Verification items for the finished model (mm, model axes). A direction names the side the tool comes from. Give positions to 0.01 mm unless a question says otherwise; leave off trailing zeros. Order: outer loops, then holes, each group sorted by start corner. A loop starts at its lowest first (then second) coordinate and runs counter-clockwise, first axis right, second up. Notation, with made-up numbers: M 71.25,34 L 87.25,34 A9 ccw 87.25,50 Z; hole C 13,-25.75 d11. An arc over 180 degrees is marked long. Answer as a JSON object with one key per item and string values.
Autodesk Inventor part; units mm, degrees
ref_plane "YZ Plane" through (0, 0, 0) normal (1, 0, 0) x (0, 1, 0)
ref_plane "XZ Plane" through (0, 0, 0) normal (0, 1, 0) x (-1, 0, 0)
ref_plane "XY Plane" through (0, 0, 0) normal (0, 0, 1) x (1, 0, 0)
sketch "Outline" plane through (0, 0, 0) normal (0, 0, 1) x (1, 0, 0)
  line L0 (0, 37.1721) -> (55.88, 37.1721) construction
  line L1 (55.88, 37.1721) -> (55.88, 115.2771) construction
  line L2 (55.88, 115.2771) -> (0, 115.2771) construction
  line L3 (0, 115.2771) -> (0, 37.1721) construction
  circle A0 centre (27.94, 115.2771) radius 26.67 construction
  circle A1 centre (27.94, 37.1721) radius 52.07 construction
  circle A2 centre (27.94, 115.2771) radius 27.94 construction
  circle A3 centre (27.94, 37.1721) radius 53.34 construction
  arc A4 (55.88, 115.2771) -> (0, 115.2771) centre (27.94, 115.2771) ccw
  line L4 (55.88, 115.2771) -> (55.88, 82.609)
  arc A5 (81.28, 37.1721) -> (55.88, 82.609) centre (27.94, 37.1721) ccw
  line L5 (142.2611, 29.5521) -> (-127.7704, 29.5521) construction
  line L6 (81.28, 37.1721) -> (81.28, 29.5521)
  line L7 (0, 29.5521) -> (81.28, 29.5521)
  line L8 (0, 115.2771) -> (0, 29.5521)
  dimension "d20" = 78.105
  dimension "d23" = 104.14
  dimension "d25" = 53.34
  dimension "d27" = 1.27
  dimension "d28" = 55.88
  dimension "d29" = 55.88
  dimension "d30" = 1.27
  dimension "d31" = 7.62
extrude "Edge Ext" add sketch "Outline" along normal blind 6.35
shell "Edge_Shell" thickness 1.5875 outward yes removed faces 1 at (18.6267, 75.8128, 6.35)
sketch "Pegs" plane through (27.94, 115.2771, 0) normal (0, 0, 1) x (1, 0, 0)
  arc A0 (53.34, -78.105) -> (27.94, -32.6681) centre (0, -78.105) ccw
  circle A1 centre (0, -78.105) radius 1.143
  point P0 (-27.94, -115.2771)
  dimension "d36" = 2.286
extrude "Pegs_Ext" add sketch "Pegs" along normal blind 7.9375
sketch "Sketch3" plane through (27.94, 115.2771, 0) normal (0, 0, 1) x (1, 0, 0)
  circle A0 centre (0, -78.105) radius 1.143
  arc A1 (27.94, 0) -> (-27.94, 0) centre (0, 0) ccw
  line L0 (-27.94, 0) -> (-27.94, -85.725)
  line L1 (-27.94, -85.725) -> (53.34, -85.725)
  line L2 (53.34, -85.725) -> (53.34, -78.105)
  arc A2 (53.34, -78.105) -> (27.94, -32.6681) centre (0, -78.105) ccw
  line L3 (27.94, -32.6681) -> (27.94, 0)
  line L4 (46.559, 0) -> (-50.3798, 0) construction
  line L5 (0, 35.3546) -> (0, -92.7907) construction
  circle A3 centre (0, 0) radius 27.94 construction
  line L6 (46.559, 3.175) -> (-50.3798, 3.175) construction
  line L7 (46.559, -3.175) -> (-50.3798, -3.175) construction
  line L8 (-27.94, 3.175) -> (27.94, 3.175)
  line L9 (27.94, 3.175) -> (27.94, -3.175)
  line L10 (27.94, -3.175) -> (-27.94, -3.175)
  line L11 (-27.94, -3.175) -> (-27.94, 3.175)
  line L12 (3.175, 35.3546) -> (3.175, -85.725) construction
  line L13 (-3.175, 35.3546) -> (-3.175, -92.7907) construction
  line L14 (-3.175, 27.94) -> (3.175, 27.94)
  line L15 (3.175, 27.94) -> (3.175, -85.725)
  line L16 (3.175, -85.725) -> (-3.175, -85.725)
  line L17 (-3.175, -85.725) -> (-3.175, 27.94)
  arc A4 (27.94, 0) -> (-27.94, 0) centre (0, 0) ccw
  line L18 (0, -78.105) -> (73.8592, -78.105) construction
  line L19 (0, -78.105) -> (-73.8592, -78.105) construction
  line L20 (71.8226, -74.93) -> (-43.3054, -74.93) construction
  line L21 (71.8226, -81.28) -> (-43.3054, -81.28) construction
  line L22 (-27.94, -74.93) -> (53.34, -74.93)
  line L23 (53.34, -74.93) -> (53.34, -81.28)
  line L24 (53.34, -81.28) -> (-27.94, -81.28)
  line L25 (-27.94, -81.28) -> (-27.94, -74.93)
  arc A5 (53.34, -78.105) -> (27.94, -32.6681) centre (0, -78.105) ccw
  line L26 (-27.94, -85.725) -> (-27.94, 0)
  point P0 (-27.94, -115.2771)
  dimension "d39" = 3.175
  dimension "d40" = 3.175
  dimension "d41" = 55.88
  dimension "d42" = 55.88
  dimension "d43" = 3.175
  dimension "d44" = 3.175
  dimension "d45" = 113.665
  dimension "d46" = 113.665
  dimension "d47" = 3.175
equation "\"d29\" = d28"
equation "\"d41\" = d42"
equation "\"d46\" = d45"
properties part number "housing"
Q1. Tool access check on faces 5 (the face through (55.88, 99, 3)), 6 (the face through (27.291, 144.797, 2.326)), 7 (the face through (57.468, 100, 2)). Record the directions out of +Z, -Z, +X, -X, +Y, -Y that give a thin tool (end or side, any length) a straight path to the whole face; none if there is none.
Resolved:
{"face 5": "+Z", "face 6": "+Z, -Z, +Y", "face 7": "+Z, -Z, +X, +Y"}
Q2. Material ranges on L1, parallel to X at y = 100, z = 5.5; L2, parallel to Z at x = 73.5, y = 61.5; L3, parallel to Y at x = 22.5, z = 0.5, recorded low to high.
Resolved:
{"L1": "x = -1.59 to 0, 55.88 to 57.47", "L2": "z = -1.59 to 0", "L3": "y = 27.96 to 29.55, 142.68 to 144.3"}
Q3. Gauge pin test, flat ends, axial feed: pin 1 Ø24.5 at (x, y) = (50, 71.5) entering from +Z; pin 2 Ø2.5 at (y, z) = (98, 4) entering from +X; pin 3 Ø5 at (x, z) = (45.5, 3.5) entering from +Y. Record the tip position at first contact, or that the pin passes through.
Resolved:
{"pin 1": "stops at z = 0", "pin 2": "stops at x = 57.47", "pin 3": "stops at y = 140.68"}
Q4. Release check for a two-part mould opening along X. For faces 1 (the face through (75.914, 63.921, 2.326)), 2 (the face through (28.554, 36.208, 3.913)), 3 (the face through (31, 74, -1.588)), 4 (the face through (31, 75, 0)) record: +X half, -X half, draft (parallel to the pull), parting line (faces both ways), or undercut.
Resolved:
{"face 1": "+X half", "face 2": "undercut", "face 3": "draft", "face 4": "undercut"}
Q5. Section check B-B on x = 33. Record the cut outline in (y, z).
Resolved:
{"outline": "M 27.96,-1.59 L 144.37,-1.59 L 144.37,6.35 L 142.76,6.35 L 142.76,0 L 29.55,0 L 29.55,6.35 L 27.96,6.35 Z"}
Q6. Section check A-A on y = 93. Record the cut outline in (x, z).
Resolved:
{"outline": "M -1.59,-1.59 L 57.47,-1.59 L 57.47,6.35 L 55.88,6.35 L 55.88,0 L 0,0 L 0,6.35 L -1.59,6.35 Z"}
